from build123d import *

# Parameters (mm, degrees)
SKETCH_R     = 0.825
PAD_DEPTH    = 0.4
POCKET_DEPTH = 7.151


with BuildPart() as part:
    # Sketch → Pad (new body, symmetric)
    with BuildSketch(Plane.XY):
        with BuildLine():
            Line((-4, 0), (-4, 2))
            Line((-4, 2), (-3.15, 2))
            Line((-3.15, 2), (-3.15, 9))
            Line((-3.15, 9), (-2.15, 10))
            Line((-2.15, 10), (2.15, 10))
            Line((2.15, 10), (3.15, 9))
            Line((3.15, 9), (3.15, 2))
            Line((3.15, 2), (4, 2))
            Line((4, 2), (4, 0))
            Line((4, 0), (3, 0))
            Line((3, 0), (3, -3.35))
            ThreePointArc((2.001176, -3.384267), (2.517143, -3.849706), (3, -3.35))
            Line((2.001176, -3.384267), (1.7, 1))
            Line((1.7, 1), (-1.7, 1))
            Line((-1.7, 1), (-2.001176, -3.384267))
            ThreePointArc((-3, -3.35), (-2.517143, -3.849706), (-2.001176, -3.384267))
            Line((-3, -3.35), (-3, 0))
            Line((-3, 0), (-4, 0))
        make_face()
        with Locations((0, 6)):
            Circle(SKETCH_R, mode=Mode.SUBTRACT)
    extrude(amount=PAD_DEPTH, both=True)

    # Sketch001 (on Face3 of Pad) → Pocket (cut, through all)
    with BuildSketch(Plane(origin=(-3.15, 0, 0), x_dir=(0, -1, 0), z_dir=(-1, 0, 0))):
        Polygon((-9, 0.4), (-9, 1), (-11, 1), (-11, -1), (-9, -1), (-9, -0.4), (-10, -0.2), (-10, 0.2), align=None)
    extrude(amount=-POCKET_DEPTH, mode=Mode.SUBTRACT)


solid = part.part
Verification items for the finished model (mm, model axes). Coordinates: 2 decimals unless noted, no trailing zeros. Loops run counter-clockwise (first coordinate to the right, second up) from the corner with the lowest first, then second, coordinate; pieces in that order, holes last. Notation, with made-up numbers: (60, -30) -> (104, -30) arc R16 ccw to (104, -14) -> close; hole circle Ø3 at (-26.75, 77.25). An arc over 180 degrees is marked (long way). Answer as CSV lines item,"result".
1) Depth check by flat-ended pin: pin 1 (1.5 mm diameter, centred on x = 0, y = 6, fed in from -Z). Enter the tip coordinate at first touch or a pass-through.
Found:
pin 1,"passes through"
2) Cross-section at A-A, the plane x = 0. Record the cut outline in (y, z) (3 decimals), then the cut area to 3 significant figures.
Found:
outline,"(1, -0.4) -> (5.175, -0.4) -> (5.175, 0.4) -> (1, 0.4) -> close; (6.825, -0.4) -> (9, -0.4) -> (10, -0.2) -> (10, 0.2) -> (9, 0.4) -> (6.825, 0.4) -> close"
area,"5.68 mm2"
3) Release check for a two-part mould opening along Y. For faces 1 (the flat face through (0, 4, -0.4)), 2 (the cylindrical face through (-0.2, 5.2, 0)), 3 (the flat face through (0, 9.5, -0.3)) record: +Y half, -Y half, draft (parallel to the pull), parting line (faces both ways), or undercut.
Found:
face 1,"draft"
face 2,"undercut"
face 3,"+Y half"
4) Thickness scan on L1, parallel to Y at x = 0, z = 0 (3 decimals); L2, parallel to X at y = 2.75, z = -0.05; L3, parallel to Y at x = 3.25, z = -0.05. Record the ranges inside material, lowest first. Write a range as from..to.
Found:
L1,"y = 1..5.175, 6.825..10"
L2,"x = -3.15..3.15"
L3,"y = 0..2"
5) Cross-section at B-B, the plane y = 6. Record the cut outline in (x, z) (3 decimals).
Found:
outline,"(-3.15, -0.4) -> (-0.825, -0.4) -> (-0.825, 0.4) -> (-3.15, 0.4) -> close; (0.825, -0.4) -> (3.15, -0.4) -> (3.15, 0.4) -> (0.825, 0.4) -> close"
6) Cross-section at D-D, the plane y = 2.5. Record the cut outline in (x, z), then the cut area to 3 significant figures.
Found:
outline,"(-3.15, -0.4) -> (3.15, -0.4) -> (3.15, 0.4) -> (-3.15, 0.4) -> close"
area,"5.04 mm2"
7) Cross-section at C-C, the plane x = 1.25. Record the cut outline in (y, z).
Found:
outline,"(1, -0.4) -> (9, -0.4) -> (10, -0.2) -> (10, 0.2) -> (9, 0.4) -> (1, 0.4) -> close"
